For this review, take the finished solid that the model builds, in its own axes (mm). A direction names the side the tool comes from. Round coordinates to 2 decimals unless told otherwise and drop trailing zeros. Order: outer loops, then holes, each group sorted by start corner. A loop starts at its lowest first (then second) coordinate and runs counter-clockwise, first axis right, second up. Notation, with made-up numbers: (26, -31.5) -> (75, -31.5) arc R20 cw to (75, -3.5) -> close; hole circle Ø6 at (12, 22.25). An arc over 180 degrees is marked (long way). Answer in a Markdown table with one row per item.
```python
from build123d import *

# Parameters (mm, degrees)
EXTRUDE_1_DEPTH     = 10
SKETCH_2_R          = 1.7
CUT_EXTRUDE_1_DEPTH = 10


with BuildPart() as part:
    # 草图1 → 凸台-拉伸1 (new body)
    with BuildSketch(Plane.XY):
        with BuildLine():
            Line((-6.5, 0), (-12.5, 0))
            Line((-12.5, 0), (-12.5, -2))
            Line((-12.5, -2), (-7.228416147, -2))
            ThreePointArc((-7.228416147, -2), (-4.554295868, -5.958891604), (-0.032245386, -7.499930682))
            ThreePointArc((-0.032245386, -7.499930682), (4.528634207, -5.9784172), (7.228416147, -2))
            Line((7.228416147, -2), (12.5, -2))
            Line((12.5, -2), (12.5, 0))
            Line((12.5, 0), (6.5, 0))
            ThreePointArc((6.5, 0), (0, -6.5), (-6.5, 0))
        make_face()
    extrude(amount=EXTRUDE_1_DEPTH)

    # 草图2 → 切除-拉伸1 (cut)
    with BuildSketch(Plane(origin=(0, 0, 0), x_dir=(1, 0, 0), z_dir=(0, 1, 0))):
        with Locations(Location((-9.5, -5, 0), (0, 0, 270))):
            Circle(SKETCH_2_R)
        with Locations(Location((9.5, -5, 0), (0, 0, 270))):
            Circle(SKETCH_2_R)
    extrude(amount=-CUT_EXTRUDE_1_DEPTH, mode=Mode.SUBTRACT)


solid = part.part
```
Q1. Take a section at C-C, the plane y = -6. Write out the cut boundary in (x, z), then the cut area to 3 significant figures.
Answer key:
| item | result |
|---|---|
| outline | (-4.5, 0) -> (-2.5, 0) -> (-2.5, 10) -> (-4.5, 10) -> close; (2.5, 0) -> (4.5, 0) -> (4.5, 10) -> (2.5, 10) -> close |
| area | 40.0 mm^2 |
Q2. Take a section at D-D, the plane z = 9.25. Write out the cut boundary in (x, y).
Answer key:
| item | result |
|---|---|
| outline | (-12.5, -2) -> (-7.23, -2) arc R7.5 ccw to (7.23, -2) -> (12.5, -2) -> (12.5, 0) -> (6.5, 0) arc R6.5 cw to (-6.5, 0) -> (-12.5, 0) -> close |
Q3. To check wall thickness, follow probe 1 along X at (y, z) = (-1.5, 5); probe 2 along Y at (x, z) = (10.75, 7.5); probe 3 along X at (y, z) = (-1.75, 3). State the ranges of each line that lie inside material, in increasing order.
Answer key:
| item | result |
|---|---|
| probe 1 | x = -12.5 to -11.2, -7.8 to -6.32, 6.32 to 7.8, 11.2 to 12.5 |
| probe 2 | y = -2 to 0 |
| probe 3 | x = -12.5 to -6.26, 6.26 to 12.5 |
Q4. Take a section at B-B, the plane x = 9.5. Write out the cut boundary in (y, z).
Answer key:
| item | result |
|---|---|
| outline | (-2, 0) -> (0, 0) -> (0, 3.3) -> (-2, 3.3) -> close; (-2, 6.7) -> (0, 6.7) -> (0, 10) -> (-2, 10) -> close |
Q5. Clearance check with flat-ended pins moving along their axes: pin 1 Ø2 at (x, y) = (-3.5, -2.5) entering from +Z; pin 2 Ø1 at (y, z) = (-5, 7.5) entering from -X; pin 3 Ø1.5 at (y, z) = (-4, 1) entering from -X; pin 4 Ø1.6 at (x, z) = (-9.5, 6) entering from -Y. State where each tip first meets the part, or that it passes through.
Answer key:
| item | result |
|---|---|
| pin 1 | passes through |
| pin 2 | stops at x = -6 |
| pin 3 | stops at x = -6.76 |
| pin 4 | stops at y = -2 |
Q6. The part is to be moulded in two halves that separate along X. For faces 3 (the face through (-11, -1, 5.8)), 4 (the face through (11, -2, 3.8)), 5 (the face through (-12.5, -1, 5)), 6 (the face through (0.1, -6.5, 4.9)), say which applies: +X half, -X half, draft (parallel to the pull), parting line (faces both ways), or undercut.
Answer key:
| item | result |
|---|---|
| face 3 | undercut |
| face 4 | draft |
| face 5 | -X half |
| face 6 | undercut |
Q7. Tool access review of faces 1 (the face through (12.5, -1, 5)), 2 (the face through (-11.1, -2, 3.8)): name each direction out of +Z, -Z, +X, -X, +Y, -Y from which nothing blocks a thin tool from reaching the whole face with its end or side.
Answer key:
| item | result |
|---|---|
| face 1 | +Z, -Z, +X, +Y, -Y |
| face 2 | +Z, -Z, -X, -Y |
Q8. Take a section at A-A, the plane z = 5. Write out the cut boundary in (x, y), then the cut area to 3 significant figures.
Answer key:
| item | result |
|---|---|
| outline | (-12.5, -2) -> (-11.2, -2) -> (-11.2, 0) -> (-12.5, 0) -> close; (-7.8, -2) -> (-7.23, -2) arc R7.5 ccw to (7.23, -2) -> (7.8, -2) -> (7.8, 0) -> (6.5, 0) arc R6.5 cw to (-6.5, 0) -> (-7.8, 0) -> close; (11.2, -2) -> (12.5, -2) -> (12.5, 0) -> (11.2, 0) -> close |
| area | 28.8 mm^2 |
